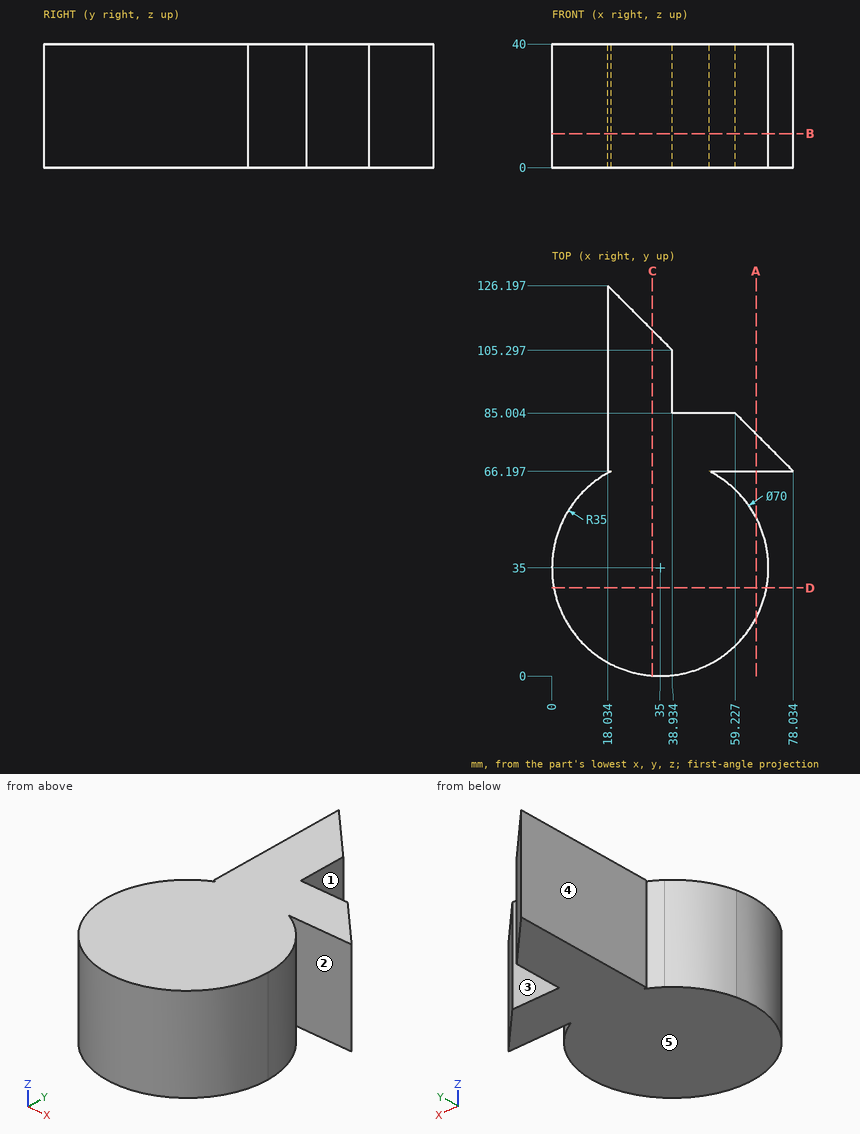
Design review of the part shown in the three views and the two pictorial views. Dimensions are in mm from the part's minimum x, y and z. A direction names the side the tool comes from. Round coordinates to 2 decimals unless told otherwise and drop trailing zeros. Order: outer loops, then holes, each group sorted by start corner. A loop starts at its lowest first (then second) coordinate and runs counter-clockwise, first axis right, second up.
(1) Take a section at D-D, the plane y = 28.5. State the section outline as (x, z) points.
Working result:
outline: (0.61, 0) - (69.39, 0) - (69.39, 40) - (0.61, 40) - close
(2) For P1, Ø20, axis at y = 99, z = 13.5, coming from the -X side; P2, Ø3, axis at x = 24, y = 60.5, coming from the -Z side; P3, Ø3, axis at y = 64, z = 21.5, coming from the +X side; P4, Ø5, axis at x = 40, z = 16.5, coming from the -Y side, all flat-tipped, find the tip position at first contact; note any pin that passes through.
Working result:
P1: stops at x = 18.03
P2: stops at z = 0
P3: stops at x = 56.65
P4: stops at y = 0.09
(3) Wall thickness on L1, parallel to Y at x = 67, z = 8 (1 decimal); L2, parallel to X at y = 99, z = 35.5; L3, parallel to Y at x = 65.5, z = 25.5 (1 decimal): over which ranges is each line inside the solid? List them lowest first.
Working result:
L1: y = 20.8 to 49.2, 66.2 to 77.2
L2: x = 18.03 to 38.93
L3: y = 17.8 to 52.2, 66.2 to 78.7
(4) Take a section at B-B, the plane z = 11. State the section outline as (x, y) points (1 decimal).
Working result:
outline: (18, 66.2) - (19.1, 66.2) arc R35 ccw (long way) to (50.9, 66.2) - (78, 66.2) - (59.2, 85) - (38.9, 85) - (38.9, 105.3) - (18, 126.2) - close
(5) Take a section at A-A, the plane x = 66. State the section outline as (y, z) points, plus the area to 3 significant figures.
Working result:
outline: (18.75, 0) - (51.25, 0) - (51.25, 40) - (18.75, 40) - close; (66.2, 0) - (78.23, 0) - (78.23, 40) - (66.2, 40) - close
area: 1,780 mm2
(6) Take a section at C-C, the plane x = 32.5. State the section outline as (y, z) points, plus the area to 3 significant figures.
Working result:
outline: (0.09, 0) - (111.73, 0) - (111.73, 40) - (0.09, 40) - close
area: 4,470 mm2
(7) Tool access review of the marked faces 4 and 5: name each direction out of +Z, -Z, +X, -X, +Y, -Y from which nothing blocks a thin tool from reaching the whole face with its end or side.
Working result:
face 4: +Z, -Z, -X, +Y
face 5: -Z, +X, -X, +Y, -Y
(8) Mouldability with a two-part tool opening along Y and no side actions: class the marked faces 1, 2 and 3 as released by +Y, released by -Y, zero draft, split by the parting line, or undercut.
Working result:
face 1: zero draft
face 2: undercut
face 3: released by +Y
